Read the model definition and answer for the solid it produces. Units are mm, in the model's axes. A direction names the side the tool comes from. Round coordinates to 2 decimals unless told otherwise and drop trailing zeros. Loops run counter-clockwise (first coordinate to the right, second up) from the corner with the lowest first, then second, coordinate; pieces in that order, holes last. Notation, with made-up numbers: (18, -8) - (25, -8) arc R20 ccw to (25, 4) - close; hole circle Ø6 at (64.5, -8). An arc over 180 degrees is marked (long way). Answer as CSV lines item,"result".
```python
from build123d import *

# Parameters (mm, degrees)
PLUNGER_STEM_START          = 24.25
SKETCH_1_R                  = 2.4
PLUNGER_STEM_DEPTH          = 10.75
PRINTABLE_FLANGE_RAMP_START = 35
SKETCH_2_R                  = 2.4
PRINTABLE_FLANGE_RAMP_DEPTH = 1.6
PRINTABLE_FLANGE_RAMP_DRAFT = -45
CAPTIVE_FLANGE_START        = 36.6
SKETCH_3_R                  = 4
CAPTIVE_FLANGE_DEPTH        = 1
EXPOSED_KEY_CAP_START       = 37.6
SKETCH_4_R                  = 2.7
EXPOSED_KEY_CAP_DEPTH       = 3.1


with BuildPart() as part:
    # 草图1 → Plunger_stem (new body)
    with BuildSketch(Plane.XY.offset(PLUNGER_STEM_START)):
        Circle(SKETCH_1_R)
    extrude(amount=PLUNGER_STEM_DEPTH)


with BuildPart() as printable_flange_ramp_tool:
    # 草图2 → Printable_flange_ramp (with draft: the straight prism first)
    with BuildSketch(Plane.XY.offset(PRINTABLE_FLANGE_RAMP_START)):
        Circle(SKETCH_2_R)
    extrude(amount=PRINTABLE_FLANGE_RAMP_DEPTH)
    # Printable_flange_ramp: the draft: its side faces are tilted about the plane it starts from
    printable_flange_ramp_sides = [printable_flange_ramp_tool.faces().sort_by_distance(p)[0] for p in [
        (-2.4, 0, 35.8),
    ]]
    draft(printable_flange_ramp_sides, Plane.XY.offset(PRINTABLE_FLANGE_RAMP_START), PRINTABLE_FLANGE_RAMP_DRAFT)


with BuildPart() as part_1:
    add(part.part)

    # Printable_flange_ramp: add printable_flange_ramp_tool
    add(printable_flange_ramp_tool.part)

    # 草图3 → Captive_flange (add)
    with BuildSketch(Plane.XY.offset(CAPTIVE_FLANGE_START)):
        Circle(SKETCH_3_R)
    extrude(amount=CAPTIVE_FLANGE_DEPTH)

    # 草图4 → Exposed_key_cap (add)
    with BuildSketch(Plane.XY.offset(EXPOSED_KEY_CAP_START)):
        Circle(SKETCH_4_R)
    extrude(amount=EXPOSED_KEY_CAP_DEPTH)


solid = part_1.part
```
1) A tool of negligible diameter and unlimited length cuts with its end or side. For faces 1 (the face through (1.29, 2.024, 29.55)), 2 (the face through (-0.867, -3.905, 37.093)), 3 (the face through (-0.585, -2.636, 39.128)), from which of +Z, -Z, +X, -X, +Y, -Y can it reach the whole face along a straight path? Write none if from no direction.
Entries:
face 1,"-Z"
face 2,"+Z, -Z"
face 3,"+Z"
2) A cutting plane is placed at A-A, the plane y = 0. Determine the outline of the cut face in (x, z), plus the area to 3 significant figures.
Entries:
outline,"(-4, 36.6) - (-2.4, 35) - (-2.4, 24.25) - (2.4, 24.25) - (2.4, 35) - (4, 36.6) - (4, 37.6) - (2.7, 37.6) - (2.7, 40.7) - (-2.7, 40.7) - (-2.7, 37.6) - (-4, 37.6) - close"
area,"86.6 mm^2"
3) Find the intervals of material crossed by line 1 (X direction, y = 1, z = 25.5); line 2 (Y direction, x = -1.5, z = 32.25); line 3 (Y direction, x = 0.75, z = 30.5), in increasing order.
Entries:
line 1,"x = -2.18 to 2.18"
line 2,"y = -1.87 to 1.87"
line 3,"y = -2.28 to 2.28"
4) A cutting plane is placed at D-D, the plane z = 36. Determine the outline of the cut face in (x, y), plus the area to 3 significant figures.
Entries:
outline,"circle Ø6.8 at (0, 0)"
area,"36.3 mm^2"
5) A cutting plane is placed at C-C, the plane z = 26. Determine the outline of the cut face in (x, y), plus the area to 3 significant figures.
Entries:
outline,"circle Ø4.8 at (0, 0)"
area,"18.1 mm^2"
6) Each of these flat-tipped pins is pushed along its axis until it touches: P1, Ø1, axis at y = 1.5, z = 38.5, coming from the +X side; P2, Ø4, axis at x = 3, z = 33.5, coming from the +Y side; P3, Ø2, axis at y = -1.5, z = 28, coming from the +X side. Where does it stop, or does it pass through?
Entries:
P1,"stops at x = 2.51"
P2,"stops at y = 2.18"
P3,"stops at x = 2.35"
